```python
from build123d import *

# Parameters (mm, degrees)
SKETCH1_W                      = 39.6875
SKETCH1_H                      = 15.875
BOSS_EXTRUDE1_DEPTH            = 50.8
F_30_0_1285_DIAMETER_HOLE1_D   = 3.2639
F_4_40_TAPPED_HOLE1_D          = 2.2606
F_4_40_TAPPED_HOLE1_DEPTH      = 9.652
F_4_40_TAPPED_HOLE1_TIP        = 0.679152758
SKETCH7_R                      = 11.1125
CUT_EXTRUDE1_DEPTH             = 67.390912641
F_4_40_TAPPED_HOLE2_AT_2_COUNT = 2
F_4_40_TAPPED_HOLE2_AT_2_PITCH = 19.074064001
F_4_40_TAPPED_HOLE2_AT_3_COUNT = 2
F_4_40_TAPPED_HOLE2_AT_3_PITCH = 26.9748
F_4_40_TAPPED_HOLE2_AT_4_COUNT = 2
F_4_40_TAPPED_HOLE2_AT_4_PITCH = 19.074064001
LPATTERN1_COUNT                = 2
LPATTERN1_PITCH                = 31.75
CUT_EXTRUDE2_REACH             = 97.567
CUT_EXTRUDE2_END_RADIUS        = 11.1125
SKETCH10_W                     = 9.4996
SKETCH10_H                     = 3.175
FILLET1_R                      = 1.5748
SKETCH11_W                     = 9.4996
SKETCH11_H                     = 6.3754
CUT_EXTRUDE3_DEPTH             = 3.175
FILLET2_R                      = 1.5748
MIRROR3_START                  = -39.6875
MIRROR3_DEPTH                  = 16.928554124
MIRROR3_2_DEPTH                = 3.175


# Read off the part's stored shape, not the designer's step: Mirror3
with BuildPart() as part:
    # Sketch1 → Boss-Extrude1 (new body)
    with BuildSketch(Plane(origin=(0, 0, 0), x_dir=(1, 0, 0), z_dir=(0, 1, 0))):
        with Locations((19.84375, 7.9375)):
            Rectangle(SKETCH1_W, SKETCH1_H)
    extrude(amount=-BOSS_EXTRUDE1_DEPTH)

    # #30 (0.1285) Diameter Hole1 (through all)
    with Locations(Plane(origin=(0, 0, 0), x_dir=(-1, 0, 0), z_dir=(0, 1, 0))):
        with Locations((-36.5125, -9.525)):
            Hole(F_30_0_1285_DIAMETER_HOLE1_D / 2)

    # #4-40 Tapped Hole1
    with Locations(Plane(origin=(39.6875, 0, 0), x_dir=(0, 0, -1), z_dir=(1, 0, 0))):
        with Locations((13.4874, -6.35), (13.4874, -34.925)):
            Hole(F_4_40_TAPPED_HOLE1_D / 2, depth=F_4_40_TAPPED_HOLE1_DEPTH)
            with Locations((0, 0, -(F_4_40_TAPPED_HOLE1_DEPTH + F_4_40_TAPPED_HOLE1_TIP / 2))):  # 118° drill point
                Cone(0, F_4_40_TAPPED_HOLE1_D / 2, F_4_40_TAPPED_HOLE1_TIP, mode=Mode.SUBTRACT)

    # Mirror1: part across plane


with BuildPart() as part_1:
    add(part.part)
    add(part.part.mirror(Plane(origin=(0, -50.8, 0), x_dir=(1, 0, 0), z_dir=(0, 0, 1))))

    # Mirror2: part across plane


with BuildPart() as part_2:
    add(part_1.part)
    add(part_1.part.mirror(Plane(origin=(0, -50.8, -15.875), x_dir=(0, 0, 1), z_dir=(-1, 0, 0))))

    # Sketch7 → Cut-Extrude1 (cut, through all)
    with BuildSketch(Plane(origin=(0, 0, 0), x_dir=(-1, 0, 0), z_dir=(0, 1, 0))):
        with Locations(Location((-19.0373, 0, 0), (0, 0, 90))):
            Circle(SKETCH7_R)
    cut_extrude1 = extrude(amount=-CUT_EXTRUDE1_DEPTH, mode=Mode.SUBTRACT)

    # Sketch8 → #4-40 Tapped Hole2 (revolve, cut)
    with BuildSketch(Plane(origin=(9.500267999, 0, -9.537032001), x_dir=(0, 0, 1), z_dir=(1, 0, 0))):
        Polygon((0, 0), (0, 10.331152758), (1.1303, 9.652), (1.1303, 0), align=None)
    f_4_40_tapped_hole2 = revolve(axis=Axis((9.500267999, 6.35, -9.537032001), (0, -1, 0)), mode=Mode.SUBTRACT)

    # #4-40 Tapped Hole2 at 2: #4-40 Tapped Hole2 ×2
    with Locations(*[(i * F_4_40_TAPPED_HOLE2_AT_2_PITCH, 0, 0) for i in range(1, F_4_40_TAPPED_HOLE2_AT_2_COUNT)]):
        add(f_4_40_tapped_hole2, mode=Mode.SUBTRACT)

    # #4-40 Tapped Hole2 at 3: #4-40 Tapped Hole2 ×2
    with Locations(*[Vector(0.7071067811865515, 0, 0.7071067811865436) * (i * F_4_40_TAPPED_HOLE2_AT_3_PITCH) for i in range(1, F_4_40_TAPPED_HOLE2_AT_3_COUNT)]):
        add(f_4_40_tapped_hole2, mode=Mode.SUBTRACT)

    # #4-40 Tapped Hole2 at 4: #4-40 Tapped Hole2 ×2
    with Locations(*[(0, 0, i * F_4_40_TAPPED_HOLE2_AT_4_PITCH) for i in range(1, F_4_40_TAPPED_HOLE2_AT_4_COUNT)]):
        add(f_4_40_tapped_hole2, mode=Mode.SUBTRACT)

    # LPattern1: Cut-Extrude1, #4-40 Tapped Hole2 ×2
    with Locations(*[(-i * LPATTERN1_PITCH, 0, 0) for i in range(1, LPATTERN1_COUNT)]):
        add(cut_extrude1, mode=Mode.SUBTRACT)
        add(f_4_40_tapped_hole2, mode=Mode.SUBTRACT)

    # LPattern1 copy 1 sketch → LPattern1 copy 1 (revolve, cut)
    with BuildSketch(Plane(origin=(-3.175667999, 0, -9.537032001), x_dir=(0, 0, 1), z_dir=(1, 0, 0))):
        Polygon((0, 0), (0, 10.331152758), (1.1303, 9.652), (1.1303, 0), align=None)
    revolve(axis=Axis((-3.175667999, 6.35, -9.537032001), (0, -1, 0)), mode=Mode.SUBTRACT)

    # LPattern1 copy 2 sketch → LPattern1 copy 2 (revolve, cut)
    with BuildSketch(Plane(origin=(-3.175667999, 0, 9.537032001), x_dir=(0, 0, 1), z_dir=(1, 0, 0))):
        Polygon((0, 0), (0, 10.331152758), (1.1303, 9.652), (1.1303, 0), align=None)
    revolve(axis=Axis((-3.175667999, 6.35, 9.537032001), (0, -1, 0)), mode=Mode.SUBTRACT)

    # LPattern1 copy 3 sketch → LPattern1 copy 3 (revolve, cut)
    with BuildSketch(Plane(origin=(-22.249732001, 0, 9.537032001), x_dir=(0, 0, 1), z_dir=(1, 0, 0))):
        Polygon((0, 0), (0, 10.331152758), (1.1303, 9.652), (1.1303, 0), align=None)
    revolve(axis=Axis((-22.249732001, 6.35, 9.537032001), (0, -1, 0)), mode=Mode.SUBTRACT)

    # Cut-Extrude2: up to this cylinder (the profile starts outside it)
    cut_extrude2_end = Plane(origin=(19.0373, -4.7625, 0), z_dir=(0, 1, 0)) * Cylinder(CUT_EXTRUDE2_END_RADIUS, 218.359, mode=Mode.PRIVATE)
    # Sketch10 → Cut-Extrude2 (cut, up to the surface)
    with BuildSketch(Plane(origin=(39.6875, 0, 0), x_dir=(0, 0, -1), z_dir=(1, 0, 0)), mode=Mode.PRIVATE) as cut_extrude2_sk1:
        with Locations((0, -4.7625)):
            Rectangle(SKETCH10_W, SKETCH10_H)
    cut_extrude2_tool1 = extrude(cut_extrude2_sk1.sketch, amount=-CUT_EXTRUDE2_REACH, mode=Mode.PRIVATE) - cut_extrude2_end
    add(cut_extrude2_tool1.solids().sort_by_distance((39.6875, -4.7625, 0))[0], mode=Mode.SUBTRACT)

    # Fillet1
    fillet1_edges = [part_2.edges().sort_by_distance(p)[0] for p in [
        (34.385522938, -6.35, 4.7498),
        (34.385522938, -3.175, 4.7498),
        (34.385522938, -3.175, -4.7498),
        (34.385522938, -6.35, -4.7498),
    ]]
    fillet(fillet1_edges, radius=FILLET1_R)

    # Sketch11 → Cut-Extrude3 (cut)
    with BuildSketch(Plane(origin=(39.6875, 0, 0), x_dir=(0, 0, -1), z_dir=(1, 0, 0))):
        with Locations((0, -7.9375)):
            Rectangle(SKETCH11_W, SKETCH11_H)
    extrude(amount=-CUT_EXTRUDE3_DEPTH, mode=Mode.SUBTRACT)

    # Fillet2
    fillet2_edges = [part_2.edges().sort_by_distance(p)[0] for p in [
        (38.1, -11.1252, -4.7498),
        (38.1, -11.1252, 4.7498),
    ]]
    fillet(fillet2_edges, radius=FILLET2_R)

    # Mirror3 outline → Mirror3 (cut)
    with BuildSketch(Plane.YZ.offset(MIRROR3_START)):
        with BuildLine():
            Line((-6.35, 3.175), (-6.35, -3.175))
            ThreePointArc((-6.35, -3.175), (-5.888751759, -4.288551759), (-4.7752, -4.7498))
            Line((-4.7752, -4.7498), (-4.7498, -4.7498))
            ThreePointArc((-4.7498, -4.7498), (-3.636248241, -4.288551759), (-3.175, -3.175))
            Line((-3.175, -3.175), (-3.175, 3.175))
            ThreePointArc((-3.175, 3.175), (-3.636248241, 4.288551759), (-4.7498, 4.7498))
            Line((-4.7498, 4.7498), (-4.7752, 4.7498))
            ThreePointArc((-4.7752, 4.7498), (-5.888751759, 4.288551759), (-6.35, 3.175))
        make_face()
    extrude(amount=MIRROR3_DEPTH, mode=Mode.SUBTRACT)

    # Mirror3 2 outline → Mirror3 2 (cut)
    with BuildSketch(Plane.YZ.offset(MIRROR3_START)):
        with BuildLine():
            ThreePointArc((-4.7752, -4.7498), (-5.888751759, -4.288551759), (-6.35, -3.175))
            Line((-6.35, -3.175), (-6.35, 3.175))
            ThreePointArc((-6.35, 3.175), (-5.888751759, 4.288551759), (-4.7752, 4.7498))
            Line((-4.7752, 4.7498), (-9.5504, 4.7498))
            ThreePointArc((-9.5504, 4.7498), (-10.663951759, 4.288551759), (-11.1252, 3.175))
            Line((-11.1252, 3.175), (-11.1252, -3.175))
            ThreePointArc((-11.1252, -3.175), (-10.663951759, -4.288551759), (-9.5504, -4.7498))
            Line((-9.5504, -4.7498), (-4.7752, -4.7498))
        make_face()
    extrude(amount=MIRROR3_2_DEPTH, mode=Mode.SUBTRACT)


solid = part_2.part
```
CAD build for the part. Positions are in the model's coordinates, mm. A direction names the side the tool comes from. Give positions to 0.01 mm unless a question says otherwise; leave off trailing zeros. Order: outer loops, then holes, each group sorted by start corner. A loop starts at its lowest first (then second) coordinate and runs counter-clockwise, first axis right, second up.
(1) Saw through at B-B, the plane z = 0. State how many separate pieces and enclosed holes the cut face has, then the cut area to 3 significant figures.
(2) Drill centre lines: L1, parallel to X at y = -25.5, z = 0.5; L2, parallel to Z at x = -32, y = -6.5 (3 decimals); L3, parallel to X at y = -30, z = 5.5. Where is each one in solid material? Low to high.
(3) Saw through at C-C, the plane y = -22. Give the cut face in (x, z) (1 decimal), then the cut area to 3 significant figures.
(4) Tool access for faces 4 (the flat face through (-38, -11.125, 0)), 5 (the cylindrical face through (8.74, -4.76, 8.7)), 6 (the flat face through (33, -6.35, 0)): list every direction of +Z, -Z, +X, -X, +Y, -Y with a clear straight run to the whole face (end or side of a thin tool).
(5) Mould opens along Y. For faces 1 (the cylindrical face through (-21.247, -4.758, -9.015)), 2 (the conical face through (28.38, -10.213, 9.511)), 3 (the cylindrical face through (-34.8, -33.8, -13.6)) say: released by +Y, released by -Y, zero draft, split by the parting line, or undercut.
(6) Flat gauge pins, fed straight in: pin 1 (6 mm diameter, centred on y = -8, z = -1, fed in from -X); pin 2 (1.4 mm diameter, centred on y = -6.35, z = 13.49, fed in from -X). Where does each tip first touch, or does it go through?
(7) Saw through at A-A, the plane x = -27.5. Give the cut face in (y, z) (3 decimals).
Results found:
1. separate pieces: 5
1. enclosed holes: 0
1. area: 1,660 mm2
2. L1: x = -39.69 to -23.81, -1.61 to 7.94, 30.14 to 39.69
2. L2: z = -15.875 to -14.608, -12.367 to 12.367, 14.608 to 15.875
2. L3: x = -39.69 to -22.37, -3.06 to 9.38, 28.69 to 39.69
3. outline: (-39.7, -15.9) - (39.7, -15.9) - (39.7, 15.9) - (-39.7, 15.9) - close; hole circle Ø3.3 at (-36.5, -9.5); hole circle Ø3.3 at (-36.5, 9.5); hole circle Ø22.2 at (-12.7, 0); hole circle Ø22.2 at (19, 0); hole circle Ø3.3 at (36.5, -9.5); hole circle Ø3.3 at (36.5, 9.5)
3. area: 1,710 mm2
4. face 4: -X
4. face 5: +Y
4. face 6: +X
5. face 1: zero draft
5. face 2: released by +Y
5. face 3: undercut
6. pin 1: stops at x = -36.51
6. pin 2: stops at x = -29.78
7. outline: (-50.8, -15.875) - (0, -15.875) - (0, 15.875) - (-50.8, 15.875) - close; hole (-6.35, -3.175) arc R1.575 ccw to (-4.775, -4.75) - (-4.75, -4.75) arc R1.575 ccw to (-3.175, -3.175) - (-3.175, 3.175) arc R1.575 ccw to (-4.75, 4.75) - (-4.775, 4.75) arc R1.575 ccw to (-6.35, 3.175) - close
